Design review of the part built by this model. Coordinates are the model's own, in mm. A direction names the side the tool comes from. Coordinates: 2 decimals unless noted, no trailing zeros. Write each loop counter-clockwise with the first axis right and the second up, starting at its lowest first coordinate (ties: lowest second). Pieces come first, ordered by that corner, then holes. Notation, with made-up numbers: (-39, -16) -> (6, -16) arc R22 cw to (6, 5) -> close; hole circle Ø2 at (-20.5, -36). An arc over 180 degrees is marked (long way). Answer in a Markdown table with one row per item. Add a question column.
Item 1: For faces 1 (the face through (0.427, 2.807, -1.923)), 2 (the face through (-1.096, 0.641, 2.107)), list the 3-axis set-ups (+Z, -Z, +X, -X, +Y, -Y) from which the entire face can be reached by the end or side of a thin tool; tool diameter is ignored.
Item 2: To check wall thickness, follow line 1 (Y direction, x = -0.65, z = 2.2); line 2 (Y direction, x = 0.45, z = 1.45); line 3 (Z direction, x = 0.05, y = 7). State the ranges of each line that lie inside material, in increasing order.
Item 3: Take a section at A-A, the plane x = -1.6. Write out the cut boundary in (y, z).
Item 4: Take a section at D-D, the plane y = 2. Write out the cut boundary in (x, z) (3 decimals), and give its area (3 significant figures).
Item 5: Take a section at C-C, the plane z = -1.5. Write out the cut boundary in (x, y).
Item 6: Clearance check with flat-ended pins moving along their axes: P1, Ø1, axis at y = 8, z = 1, coming from the +X side; P2, Ø1.5, axis at x = -0.5, y = 8.5, coming from the -Z side; P3, Ø1, axis at x = 0, y = 7.5, coming from the +Z side. State where each tip first meets the part, or that it passes through.
Item 7: Take a section at B-B, the plane y = 4.25. Write out the cut boundary in (x, z), and give its area (3 significant figures).
Autodesk Inventor part; units mm, degrees
ref_plane "YZ Plane" through (0, 0, 0) normal (1, 0, 0) x (0, 1, 0)
ref_plane "XZ Plane" through (0, 0, 0) normal (0, 1, 0) x (-1, 0, 0)
ref_plane "XY Plane" through (0, 0, 0) normal (0, 0, 1) x (1, 0, 0)
sketch "Sketch1" plane through (0, 0, 0) normal (0, 0, 1) x (1, 0, 0)
  line L0 (0, 0) -> (-2.375, 0)
  line L1 (-1.97, 2.3) -> (-1.97, 3.3)
  line L2 (-1.97, 3.3) -> (-1.78, 3.3)
  line L3 (-1.78, 3.3) -> (-1.78, 7.87)
  line L4 (-1.78, 7.87) -> (-1.17, 7.87)
  line L5 (-1.17, 7.87) -> (-1.17, 9.9224)
  arc A0 (0, 10.16) -> (-1.17, 9.9224) centre (0, 7.16) ccw
  line L6 (0, 0) -> (0, 10.16)
  line L7 (-1.97, 2.3) -> (-2.005, 2.3)
  line L8 (-2.005, 2.3) -> (-2.005, 1.3)
  line L9 (-2.005, 1.3) -> (-2.375, 1.3)
  line L10 (-2.375, 1.3) -> (-2.375, 0)
  dimension "d0" = 1.17
  dimension "d1" = 1.78
  dimension "d2" = 1.97
  dimension "d3" = 2.005
  dimension "d4" = 2.375
  dimension "d5" = 1.3
  dimension "d6" = 7.87
  dimension "d7" = 2.29
  dimension "d8" = 1
  dimension "d9" = 1
  dimension "d10" = 3
revolve "Revolution1" add sketch "Sketch1" angle 360 about axis through (0, 0, 0) along (0, 1, 0)
properties part number "0871 Spring Loaded"
Answers:
| question | item | result |
|---|---|---|
| 1 | face 1 | +Y |
| 1 | face 2 | +Y, -Y |
| 2 | line 1 | y = 0 to 1.3 |
| 2 | line 2 | y = 0 to 7.87 |
| 2 | line 3 | z = -1.78 to 1.78 |
| 3 | outline | (0, -1.76) -> (1.3, -1.76) -> (1.3, -1.21) -> (2.3, -1.21) -> (2.3, -1.15) -> (3.3, -1.15) -> (3.3, -0.78) -> (7.87, -0.78) -> (7.87, 0.78) -> (3.3, 0.78) -> (3.3, 1.15) -> (2.3, 1.15) -> (2.3, 1.21) -> (1.3, 1.21) -> (1.3, 1.76) -> (0, 1.76) -> close |
| 4 | outline | circle Ø4.01 at (0, 0) |
| 4 | area | 12.6 mm^2 |
| 5 | outline | (-1.84, 0) -> (1.84, 0) -> (1.84, 1.3) -> (1.33, 1.3) -> (1.33, 2.3) -> (1.28, 2.3) -> (1.28, 3.3) -> (0.96, 3.3) -> (0.96, 7.87) -> (-0.96, 7.87) -> (-0.96, 3.3) -> (-1.28, 3.3) -> (-1.28, 2.3) -> (-1.33, 2.3) -> (-1.33, 1.3) -> (-1.84, 1.3) -> close |
| 6 | P1 | stops at x = 1.7 |
| 6 | P2 | stops at z = -1.78 |
| 6 | P3 | stops at z = 1.78 |
| 7 | outline | circle Ø3.56 at (0, 0) |
| 7 | area | 9.95 mm^2 |
